Can you work these out from the model? Positions are in its coordinate system, mm. A direction names the side the tool comes from. Coordinates: 2 decimals unless noted, no trailing zeros. Loops run counter-clockwise (first coordinate to the right, second up) from the corner with the lowest first, then second, coordinate; pieces in that order, holes last.
```python
from build123d import *

# Parameters (mm, degrees)
BOSS_EXTRUDE1_DEPTH = 10
SKETCH2_R           = 4
BOSS_EXTRUDE2_DEPTH = 6
SKETCH3_R           = 0.5
BOSS_EXTRUDE3_DEPTH = 5
SKETCH4_R           = 1.701881869
BOSS_EXTRUDE4_DEPTH = 2


with BuildPart() as part:
    # Sketch1 → Boss-Extrude1 (new body)
    with BuildSketch(Plane(origin=(0, 0, 0), x_dir=(1, 0, 0), z_dir=(0, 1, 0))):
        Polygon((0, 0), (14.878679656, 0), (17, -2.121320344), (17, -17), (22, -17), (22, -19), (17, -19), (17, -23), (0, -23), (0, -19), (-5, -19), (-5, -17), (0, -17), align=None)
    extrude(amount=BOSS_EXTRUDE1_DEPTH)

    # Sketch2 → Boss-Extrude2 (add)
    with BuildSketch(Plane.XY.offset(23)):
        with Locations((12, 5)):
            Circle(SKETCH2_R)
    extrude(amount=BOSS_EXTRUDE2_DEPTH)

    # Sketch3 → Boss-Extrude3 (add)
    with BuildSketch(Plane.XY.offset(29)):
        with Locations((12, 5)):
            Circle(SKETCH3_R)
    extrude(amount=BOSS_EXTRUDE3_DEPTH)

    # Sketch4 → Boss-Extrude4 (add)
    with BuildSketch(Plane(origin=(0, 0, 0), x_dir=(-1, 0, 0), z_dir=(0, 0, -1))):
        with Locations((-11.878679656, 5)):
            Circle(SKETCH4_R)
    extrude(amount=BOSS_EXTRUDE4_DEPTH)


solid = part.part
```
Item 1: Suppose I cut it at A-A, the plane y = 9.5. Please give me the cut outline in (x, z).
Results are:
outline: (-5, 17) - (0, 17) - (0, 0) - (14.88, 0) - (17, 2.12) - (17, 17) - (22, 17) - (22, 19) - (17, 19) - (17, 23) - (0, 23) - (0, 19) - (-5, 19) - close
Item 2: Suppose I cut it at B-B, the plane x = 12. Please give me the cut outline in (y, z).
Results are:
outline: (0, 0) - (3.3, 0) - (3.3, -2) - (6.7, -2) - (6.7, 0) - (10, 0) - (10, 23) - (9, 23) - (9, 29) - (5.5, 29) - (5.5, 34) - (4.5, 34) - (4.5, 29) - (1, 29) - (1, 23) - (0, 23) - close
Item 3: I'm going to push flat-ended pins straight in: P1, Ø2.5, axis at x = 10.5, y = 3.5, coming from the +Z side; P2, Ø4, axis at x = -2.5, y = 4, coming from the +Z side; P3, Ø3, axis at x = 4, y = 8.5, coming from the +Z side. Where does each tip first touch, or does it pass through?
Results are:
P1: stops at z = 29
P2: stops at z = 19
P3: stops at z = 23
Item 4: I need wall thicknesses on line 1 along Z through (x, y) = (5.25, 3.5); line 2 along X through (y, z) = (6.5, 6); line 3 along Z through (x, y) = (-2, 9.5). Which ranges of each line are inside material? Lowest first, please.
Results are:
line 1: z = 0 to 23
line 2: x = 0 to 17
line 3: z = 17 to 19
Item 5: On a 3-axis mill with a long thin cutter (end or side, diameter ignored), from which of +Z, -Z, +X, -X, +Y, -Y can I reach the whole of each face in a straight line? I mean faces 1 (the face through (11.935, 5.496, 31.465)), 2 (the face through (19, 5, 17)), 3 (the face through (0, 5, 21)). Say none if no direction works.
Results are:
face 1: +Z
face 2: -Z, +X, +Y, -Y
face 3: +Z, -X, +Y, -Y
Item 6: Suppose I cut it at C-C, the plane z = 15.5. Please give me the cut outline in (x, y).
Results are:
outline: (0, 0) - (17, 0) - (17, 10) - (0, 10) - close
Item 7: Suppose I cut it at D-D, the plane y = 5. Please give me the cut outline in (x, z), plus the area to 3 significant figures.
Results are:
outline: (-5, 17) - (0, 17) - (0, 0) - (10.18, 0) - (10.18, -2) - (13.58, -2) - (13.58, 0) - (14.88, 0) - (17, 2.12) - (17, 17) - (22, 17) - (22, 19) - (17, 19) - (17, 23) - (16, 23) - (16, 29) - (12.5, 29) - (12.5, 34) - (11.5, 34) - (11.5, 29) - (8, 29) - (8, 23) - (0, 23) - (0, 19) - (-5, 19) - close
area: 469 mm2
